Drawing for the job (mm, zero at the part's lowest x, y, z). Round coordinates to 2 decimals unless told otherwise and drop trailing zeros. Write each loop counter-clockwise with the first axis right and the second up, starting at its lowest first coordinate (ties: lowest second). Pieces come first, ordered by that corner, then holes.
Item 1: Band-saw the part on B-B, the plane y = 16.25. Write the cut outline in (x, z).
Item 2: Drop flat-ended pins along their axis: pin 1 Ø4 at (x, y) = (14, 45) entering from +Z; pin 2 Ø12 at (x, y) = (14.5, 32) entering from +Z; pin 3 Ø3 at (y, z) = (60.5, 26.5) entering from +X. Give the stop position or say it passes through.
Item 3: Wall check: probe 1 along Y at (x, z) = (11, 15); probe 2 along Y at (x, z) = (15.75, 14.25); probe 3 along Z at (x, y) = (13, 16.25). Give the ranges that are in metal, low to high.
Item 4: Mould opens along Y. For the marked faces 1, 2, 3 and 4 say: +Y half, -Y half, draft (parallel to the pull), parting line (faces both ways), or undercut.
Item 5: Band-saw the part on D-D, the plane x = 13. Write the cut outline in (y, z).
Item 6: Band-saw the part on A-A, the plane z = 15. Write the cut outline in (x, y).
Item 7: Band-saw the part on C-C, the plane z = 20. Write the cut outline in (x, y), then the cut area to 3 significant figures.
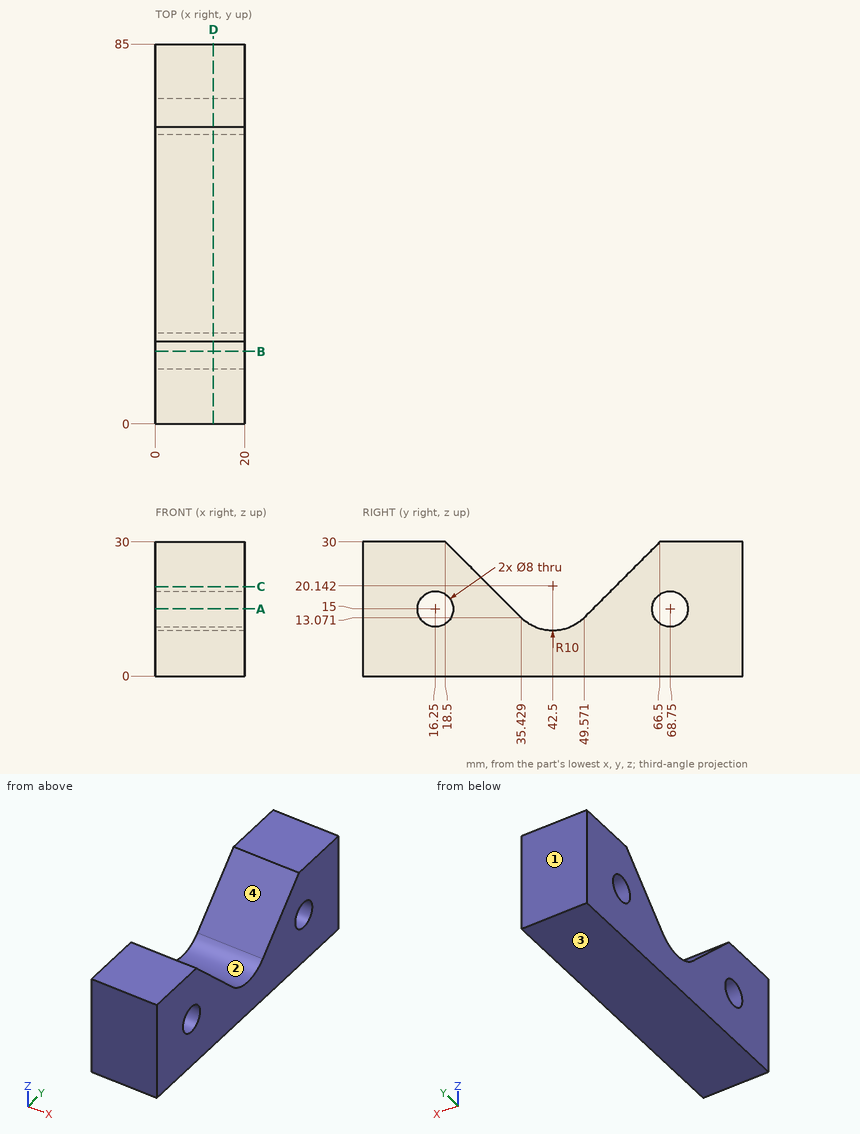
Results:
1. outline: (0, 0) - (20, 0) - (20, 11) - (0, 11) - close; (0, 19) - (20, 19) - (20, 30) - (0, 30) - close
2. pin 1: stops at z = 11.21
2. pin 2: stops at z = 22.5
2. pin 3: passes through
3. probe 1: y = 0 to 12.25, 20.25 to 33.5, 51.5 to 64.75, 72.75 to 85
3. probe 2: y = 0 to 12.32, 20.18 to 34.25, 50.75 to 64.82, 72.68 to 85
3. probe 3: z = 0 to 11, 19 to 30
4. face 1: +Y half
4. face 2: undercut
4. face 3: draft
4. face 4: undercut
5. outline: (0, 0) - (85, 0) - (85, 30) - (66.5, 30) - (49.57, 13.07) arc R10 cw to (35.43, 13.07) - (18.5, 30) - (0, 30) - close; hole circle Ø8 at (16.25, 15); hole circle Ø8 at (68.75, 15)
6. outline: (0, 0) - (20, 0) - (20, 12.25) - (0, 12.25) - close; (0, 20.25) - (20, 20.25) - (20, 33.5) - (0, 33.5) - close; (0, 51.5) - (20, 51.5) - (20, 64.75) - (0, 64.75) - close; (0, 72.75) - (20, 72.75) - (20, 85) - (0, 85) - close
7. outline: (0, 0) - (20, 0) - (20, 28.5) - (0, 28.5) - close; (0, 56.5) - (20, 56.5) - (20, 85) - (0, 85) - close
7. area: 1,140 mm2
